Design review of the part built by this model. Coordinates are the model's own, in mm. A direction names the side the tool comes from. Give positions to 0.01 mm unless a question says otherwise; leave off trailing zeros. Loops run counter-clockwise (first coordinate to the right, second up) from the corner with the lowest first, then second, coordinate; pieces in that order, holes last. Notation, with made-up numbers: M 84,-4.5 L 115,-4.5 A15 cw 115,22.5 Z; hole C 55,-30.75 d10. An arc over 180 degrees is marked long. Use a Markdown table: item, result. Add a question column.
(1) Add section A-A, the plane x = 21.5. Give the boundary of the cut face in (y, z).
(2) Add section C-C, the plane x = -10. Give the boundary of the cut face in (y, z).
(3) For faces 1 (the face through (26.85, -14, 12)), 2 (the face through (45, 9, 12)), 3 (the face through (-14, -3.15, 12)), 4 (the face through (-12.5, 4, 12)), 5 (the face through (6, 6, 25)), list the 3-axis set-ups (+Z, -Z, +X, -X, +Y, -Y) from which the entire face can be reached by the end or side of a thin tool; tool diameter is ignored.
(4) For probe 1 along Y at (x, z) = (-10, 18.25); probe 2 along Y at (x, z) = (24, 1.5); probe 3 along Y at (x, z) = (-7.5, 14.75), list the stretches that pass through material, from the lowest coordinate up.
(5) Add section D-D, the plane z = 22.5. State how many separate pieces and enclosed holes the cut face has, then the cut area to 3 significant figures.
(6) Add section B-B, the plane y = 10. Give the boundary of the cut face in (x, z), then the cut area to 3 significant figures.
(7) Draft analysis for pull direction Y (two halves, no side actions). For faces 6 (the face through (39, -15, 12)), 7 (the face through (-10, -5.5, 12)), 8 (the face through (26.85, 14, 12)), state which applies: pulls with the +Y half, pulls with the -Y half, needs draft (parallel to the pull), parting line crosses it, or undercut.
```python
from build123d import *

# Parameters (mm, degrees)
F0_R     = 3
F0_R_2   = 2.5
F1_DEPTH = 25


with BuildPart() as f1:
    # F0 (on Top) → F1 (new body)
    with BuildSketch(Plane.XY):
        with BuildLine():
            ThreePointArc((-14.5, 15), (-14.853553, 14.853553), (-15, 14.5))
            Line((-15, 14.5), (-15, 3.15))
            Line((-15, 3.15), (-12.5, 3.15))
            Line((-12.5, 3.15), (-12.5, 5.5))
            Line((-12.5, 5.5), (-6.90098, 5.5))
            ThreePointArc((-6.90098, 5.5), (-5.126404, 3.000613), (-4.5, 0))
            ThreePointArc((-4.5, 0), (-5.126404, -3.000613), (-6.90098, -5.5))
            Line((-6.90098, -5.5), (-12.5, -5.5))
            Line((-12.5, -5.5), (-12.5, -3.15))
            Line((-12.5, -3.15), (-15, -3.15))
            Line((-15, -3.15), (-15, -14.5))
            ThreePointArc((-15, -14.5), (-14.853553, -14.853553), (-14.5, -15))
            Line((-14.5, -15), (-3.15, -15))
            Line((-3.15, -15), (-3.15, -12.5))
            Line((-3.15, -12.5), (-5.5, -12.5))
            Line((-5.5, -12.5), (-5.5, -6.90098))
            ThreePointArc((-5.5, -6.90098), (-3.000613, -5.126404), (0, -4.5))
            ThreePointArc((0, -4.5), (3.000613, -5.126404), (5.5, -6.90098))
            Line((5.5, -6.90098), (5.5, -12.5))
            Line((5.5, -12.5), (3.15, -12.5))
            Line((3.15, -12.5), (3.15, -15))
            Line((3.15, -15), (26.85, -15))
            Line((26.85, -15), (26.85, -12.5))
            Line((26.85, -12.5), (24.5, -12.5))
            Line((24.5, -12.5), (24.5, -6.90098))
            ThreePointArc((24.5, -6.90098), (26.999387, -5.126404), (30, -4.5))
            ThreePointArc((30, -4.5), (33.000613, -5.126404), (35.5, -6.90098))
            Line((35.5, -6.90098), (35.5, -12.5))
            Line((35.5, -12.5), (33.15, -12.5))
            Line((33.15, -12.5), (33.15, -15))
            Line((33.15, -15), (44.5, -15))
            ThreePointArc((44.5, -15), (44.853553, -14.853553), (45, -14.5))
            Line((45, -14.5), (45, -3.15))
            Line((45, -3.15), (42.5, -3.15))
            Line((42.5, -3.15), (42.5, -5.5))
            Line((42.5, -5.5), (36.90098, -5.5))
            ThreePointArc((36.90098, -5.5), (35.126404, -3.000613), (34.5, 0))
            ThreePointArc((34.5, 0), (35.126404, 3.000613), (36.90098, 5.5))
            Line((36.90098, 5.5), (42.5, 5.5))
            Line((42.5, 5.5), (42.5, 3.15))
            Line((42.5, 3.15), (45, 3.15))
            Line((45, 3.15), (45, 14.5))
            ThreePointArc((45, 14.5), (44.853553, 14.853553), (44.5, 15))
            Line((44.5, 15), (33.15, 15))
            Line((33.15, 15), (33.15, 12.5))
            Line((33.15, 12.5), (35.5, 12.5))
            Line((35.5, 12.5), (35.5, 6.90098))
            ThreePointArc((35.5, 6.90098), (33.000613, 5.126404), (30, 4.5))
            ThreePointArc((30, 4.5), (26.999387, 5.126404), (24.5, 6.90098))
            Line((24.5, 6.90098), (24.5, 12.5))
            Line((24.5, 12.5), (26.85, 12.5))
            Line((26.85, 12.5), (26.85, 15))
            Line((26.85, 15), (3.15, 15))
            Line((3.15, 15), (3.15, 12.5))
            Line((3.15, 12.5), (5.5, 12.5))
            Line((5.5, 12.5), (5.5, 6.90098))
            ThreePointArc((5.5, 6.90098), (3.000613, 5.126404), (0, 4.5))
            ThreePointArc((0, 4.5), (-3.000613, 5.126404), (-5.5, 6.90098))
            Line((-5.5, 6.90098), (-5.5, 12.5))
            Line((-5.5, 12.5), (-3.15, 12.5))
            Line((-3.15, 12.5), (-3.15, 15))
            Line((-3.15, 15), (-14.5, 15))
        make_face()
        with Locations((-10, -10)):
            Circle(F0_R, mode=Mode.SUBTRACT)
        with Locations((40, -10)):
            Circle(F0_R, mode=Mode.SUBTRACT)
        Circle(F0_R_2, mode=Mode.SUBTRACT)
        with Locations((-10, 10)):
            Circle(F0_R, mode=Mode.SUBTRACT)
        with BuildLine():
            ThreePointArc((6.618512, -5.223944), (5.049778, -2.818585), (4.5, 0))
            ThreePointArc((4.5, 0), (5.049778, 2.818585), (6.618512, 5.223944))
            ThreePointArc((6.618512, 5.223944), (6.827677, 5.544658), (6.90098, 5.92047))
            Line((6.90098, 5.92047), (6.90098, 11.5))
            ThreePointArc((6.90098, 11.5), (7.193874, 12.207107), (7.90098, 12.5))
            Line((7.90098, 12.5), (15, 12.5))
            Line((15, 12.5), (22.09902, 12.5))
            ThreePointArc((22.09902, 12.5), (22.806126, 12.207107), (23.09902, 11.5))
            Line((23.09902, 11.5), (23.09902, 5.92047))
            ThreePointArc((23.09902, 5.92047), (23.172323, 5.544658), (23.381488, 5.223944))
            ThreePointArc((23.381488, 5.223944), (24.950222, 2.818585), (25.5, 0))
            ThreePointArc((25.5, 0), (24.950222, -2.818585), (23.381488, -5.223944))
            ThreePointArc((23.381488, -5.223944), (23.172323, -5.544658), (23.09902, -5.92047))
            Line((23.09902, -5.92047), (23.09902, -11.5))
            ThreePointArc((23.09902, -11.5), (22.806126, -12.207107), (22.09902, -12.5))
            Line((22.09902, -12.5), (15, -12.5))
            Line((15, -12.5), (7.90098, -12.5))
            ThreePointArc((7.90098, -12.5), (7.193874, -12.207107), (6.90098, -11.5))
            Line((6.90098, -11.5), (6.90098, -5.92047))
            ThreePointArc((6.90098, -5.92047), (6.827677, -5.544658), (6.618512, -5.223944))
        make_face(mode=Mode.SUBTRACT)
        with Locations((30, 0)):
            Circle(F0_R_2, mode=Mode.SUBTRACT)
        with Locations((40, 10)):
            Circle(F0_R, mode=Mode.SUBTRACT)
    extrude(amount=F1_DEPTH)


solid = f1.part
```
Established:
| question | item | result |
|---|---|---|
| 1 | outline | M -15,0 L -12.5,0 L -12.5,25 L -15,25 Z; M 12.5,0 L 15,0 L 15,25 L 12.5,25 Z |
| 2 | outline | M -15,0 L -13,0 L -13,25 L -15,25 Z; M -7,0 L -5.5,0 L -5.5,25 L -7,25 Z; M 5.5,0 L 7,0 L 7,25 L 5.5,25 Z; M 13,0 L 15,0 L 15,25 L 13,25 Z |
| 3 | face 1 | +Z, -Z, -Y |
| 3 | face 2 | +Z, -Z, +X, +Y, -Y |
| 3 | face 3 | +Z, -Z, -X |
| 3 | face 4 | +Z, -Z |
| 3 | face 5 | +Z, +X, -X, +Y, -Y |
| 4 | probe 1 | -15 to -13, -7 to -5.5, 5.5 to 7, 13 to 15 |
| 4 | probe 2 | -15 to -4.5, 4.5 to 15 |
| 4 | probe 3 | -15 to -11.66, -8.34 to -5.5, 5.5 to 8.34, 11.66 to 15 |
| 5 | separate pieces | 1 |
| 5 | enclosed holes | 7 |
| 5 | area | 633 mm^2 |
| 6 | outline | M -15,0 L -13,0 L -13,25 L -15,25 Z; M -7,0 L -5.5,0 L -5.5,25 L -7,25 Z; M 5.5,0 L 6.9,0 L 6.9,25 L 5.5,25 Z; M 23.1,0 L 24.5,0 L 24.5,25 L 23.1,25 Z; M 35.5,0 L 37,0 L 37,25 L 35.5,25 Z; M 43,0 L 45,0 L 45,25 L 43,25 Z |
| 6 | area | 245 mm^2 |
| 7 | face 6 | pulls with the -Y half |
| 7 | face 7 | undercut |
| 7 | face 8 | needs draft |
